Could you check a few things on this model? Use its own coordinates, in mm. A direction names the side the tool comes from. Round coordinates to 2 decimals unless told otherwise and drop trailing zeros. Loops run counter-clockwise (first coordinate to the right, second up) from the corner with the lowest first, then second, coordinate; pieces in that order, holes last. Notation, with made-up numbers: (15.5, 86.5) -> (67.5, 86.5) arc R29 ccw to (67.5, 120.5) -> close; hole circle Ø10 at (-33.75, -17.5). An arc over 180 degrees is marked (long way). One line per item, written item: value.
Solid Edge part; units mm, degrees
sketch "Sketch1" plane through (0, 0, 0) normal (0, 0, 1) x (1, 0, 0)
  line L0 (0, 0) -> (0, 15)
  line L1 (0, 15) -> (65, 15)
  line L2 (65, 15) -> (65, 0)
  line L3 (65, 0) -> (0, 0)
  dimension "D1" = 65
extrude "Protrusion1" add sketch "Sketch1" along normal blind 55
sketch "Sketch2" plane through (65, 7.5, 27.5) normal (1, 0, 0) x (0, 0, -1)
  line L0 (-22.5, 7.5) -> (-22.5, -7.5)
  line L1 (-22.5, -7.5) -> (22.5, -7.5)
  line L2 (22.5, -7.5) -> (22.5, 7.5)
  line L3 (22.5, 7.5) -> (-22.5, 7.5)
  dimension "D1" = 22.5
extrude "ExtrudedCutout_1" cut sketch "Sketch2" against normal blind 55
hole "Hål_till_pedal" at (57, 7.5, 55) direction (0, 0, -1) diameter 6 end through all
hole "Hål_till_kolvstång" at (0, 7.5, 27.5) direction (1, 0, 0) diameter 6 depth 5
properties material "Aluminum, 1060"
(1) For pin 1 Ø4 at (y, z) = (9.5, 38) entering from +X; pin 2 Ø3.5 at (y, z) = (7.5, 27.5) entering from -X, each with a flat end and sliding along its axis, tell me the tip position at first contact or that it passes through.
Results below:
pin 1: stops at x = 10
pin 2: stops at x = 5
(2) Please list where these lines run through material, in increasing order: L1, parallel to X at y = 7.5, z = 3.3; L2, parallel to Z at x = 43, y = 13; L3, parallel to Y at x = 2.95, z = 27.5.
Results below:
L1: x = 0 to 54, 60 to 65
L2: z = 0 to 5, 50 to 55
L3: y = 0 to 4.5, 10.5 to 15
(3) Imagine slicing it at D-D on y = 11.5. Write out the boundary of the cut face in (x, z).
Results below:
outline: (0, 0) -> (65, 0) -> (65, 5) -> (10, 5) -> (10, 50) -> (65, 50) -> (65, 55) -> (0, 55) -> close
(4) Imagine slicing it at C-C on z = 27.5. Write out the boundary of the cut face in (x, y).
Results below:
outline: (0, 0) -> (10, 0) -> (10, 15) -> (0, 15) -> (0, 10.5) -> (5, 10.5) -> (5, 4.5) -> (0, 4.5) -> close
(5) Imagine slicing it at A-A on x = 57. Write out the boundary of the cut face in (y, z), then the cut area to 3 significant figures.
Results below:
outline: (0, 0) -> (4.5, 0) -> (4.5, 5) -> (0, 5) -> close; (0, 50) -> (4.5, 50) -> (4.5, 55) -> (0, 55) -> close; (10.5, 0) -> (15, 0) -> (15, 5) -> (10.5, 5) -> close; (10.5, 50) -> (15, 50) -> (15, 55) -> (10.5, 55) -> close
area: 90.0 mm²
(6) We'd pull the mould along Y, two halves only. Please class faces 4 (the face through (33, 8, 0)), 5 (the face through (8, 15, 27)), 6 (the face through (2.5, 7.4, 24.5)): +Y half, -Y half, draft (parallel to the pull), parting line (faces both ways), or undercut.
Results below:
face 4: draft
face 5: +Y half
face 6: undercut
(7) On a 3-axis mill with a long thin cutter (end or side, diameter ignored), from which of +Z, -Z, +X, -X, +Y, -Y can I reach the whole of each face in a straight line? I mean faces 1 (the face through (59.974, 7.891, 2.535)), 2 (the face through (5, 7, 27)), 3 (the face through (10, 7, 27)). Say none if no direction works.
Results below:
face 1: +Z, -Z
face 2: -X
face 3: +X, +Y, -Y
(8) Imagine slicing it at B-B on y = 7.5. Write out the boundary of the cut face in (x, z).
Results below:
outline: (0, 0) -> (54, 0) -> (54, 5) -> (10, 5) -> (10, 50) -> (54, 50) -> (54, 55) -> (0, 55) -> (0, 30.5) -> (5, 30.5) -> (5, 24.5) -> (0, 24.5) -> close; (60, 0) -> (65, 0) -> (65, 5) -> (60, 5) -> close; (60, 50) -> (65, 50) -> (65, 55) -> (60, 55) -> close
